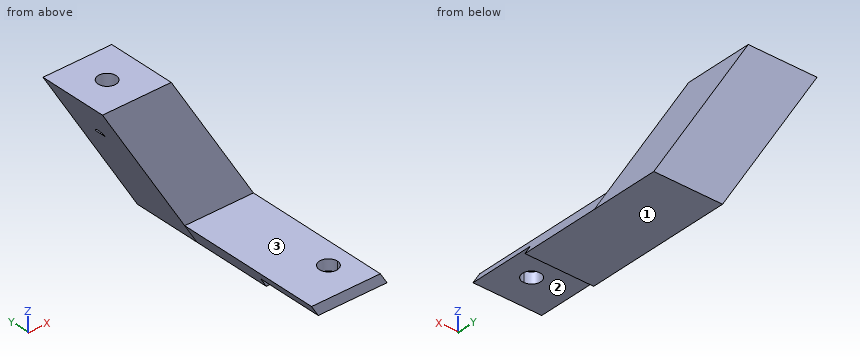
```python
from build123d import *

# Parameters (mm, degrees)
F1_DEPTH = 19.05
F3_DEPTH = 40.64
F4_R     = 2.496566
F5_DEPTH = 12.7
F7_DEPTH = 43.181
F9_DEPTH = 18.415


with BuildPart() as f1:
    # F0 (on Front) → F1 (new body)
    with BuildSketch(Plane.XZ):
        Polygon((19.05, 43.18), (0, 43.18), (26.162, 0), (35.687, 0), (45.212, 0), align=None)
    extrude(amount=F1_DEPTH)

    # F2 (on face) → F3 (join)
    with BuildSketch(Plane.XZ.offset(19.05)):
        Polygon((41.8263294118, 5.588), (22.7763294118, 5.588), (26.162, 0), (45.212, 0), align=None)
    extrude(amount=F3_DEPTH)

    # F4 (on face) → F5 (cut)
    with BuildSketch(Plane.XY.offset(43.18)):
        with Locations((9.525, -9.525)):
            Circle(F4_R)
    extrude(amount=-F5_DEPTH, mode=Mode.SUBTRACT)

    # F6 (on face) → F7 (cut, through all)
    with BuildSketch(Plane(origin=(0, 0, 0), x_dir=(1, 0, 0), z_dir=(0, 0, -1))):
        with BuildLine():
            ThreePointArc((38.186995, 50.165), (37.4547634174, 51.9327634174), (35.687, 52.664995))
            ThreePointArc((35.687, 52.664995), (33.9192365826, 48.3972365826), (38.186995, 50.165))
        make_face()
    extrude(amount=-F7_DEPTH, mode=Mode.SUBTRACT)

    # F8 (on face) → F9 (cut)
    with BuildSketch(Plane.XZ.offset(59.69)):
        Polygon((43.6730588235, 2.54), (24.6230588235, 2.54), (26.162, 0), (45.212, 0), align=None)
    extrude(amount=-F9_DEPTH, mode=Mode.SUBTRACT)


solid = f1.part
```
Model file for the job. Use its own axes, mm. Face numbers are marked on the shaded views. A direction names the side the tool comes from. Give positions to 0.01 mm unless a question says otherwise; leave off trailing zeros. Loops run counter-clockwise (first coordinate to the right, second up) from the corner with the lowest first, then second, coordinate; pieces in that order, holes last. Notation, with made-up numbers: M 68.25,29.25 L 105.25,29.25 A15 ccw 105.25,42.25 Z; hole C 3.5,-35 d9. An arc over 180 degrees is marked long. Use one line per item in the form item = value.
Item 1: Flat gauge pins, fed straight in: pin 1 Ø9.5 at (x, y) = (36, -47.5) entering from +Z; pin 2 Ø1.3 at (x, y) = (10.5, -10) entering from +Z; pin 3 Ø6 at (x, y) = (29.5, -52) entering from -Z. Where does each tip first touch, or does it go through?
Filled in:
pin_1 = 5.59
pin_2 = 30.48
pin_3 = 2.54
Item 2: Drill centre lines: L1, parallel to Z at x = 39, y = -24; L2, parallel to Y at x = 24, z = 6.5; L3, parallel to Y at x = 36, z = 4.5. Where is each one in solid material? Low to high.
Filled in:
L1 = 0 to 5.59
L2 = -19.05 to 0
L3 = -59.69 to -52.65, -47.68 to 0
Item 3: Slice it at C-C on x = 41. List the corners of the cut face in (y, z) (3 decimals), and give its area (3 significant figures).
Filled in:
outline = M -59.69,2.54 L -41.275,2.54 L -41.275,0 L 0,0 L 0,6.952 L -19.05,6.952 L -19.05,5.588 L -59.69,5.588 Z
area = 313 mm^2
Item 4: Slice it at D-D on z = 21. List the corners of the cut face in (x, y), and give its area (3 significant figures).
Filled in:
outline = M 13.44,-19.05 L 32.49,-19.05 L 32.49,0 L 13.44,0 Z
area = 363 mm^2
Item 5: Slice it at B-B on y = -56. List the corners of the cut face in (x, z).
Filled in:
outline = M 22.78,5.59 L 24.62,2.54 L 43.67,2.54 L 41.83,5.59 Z
Item 6: Which spindle directions (+Z, -Z, +X, -X, +Y, -Y) get a long thin tool onto all of the face, cutting with end or side? Do the marked faces 1, 2 and 3. Say none if no direction does.
Filled in:
face_1 = -Z, +X, -X, +Y, -Y
face_2 = -Z, +X, -X, -Y
face_3 = +Z, +X, -X, -Y
Item 7: Slice it at A-A on x = 34. List the corners of the cut face in (y, z) (3 decimals).
Filled in:
outline = M -59.69,2.54 L -52.01,2.54 L -52.01,5.588 L -59.69,5.588 Z; M -48.32,2.54 L -41.275,2.54 L -41.275,0 L 0,0 L 0,18.505 L -19.05,18.505 L -19.05,5.588 L -48.32,5.588 Z
